from build123d import *

# Parameters (mm, degrees)
SKETCH1_R               = 13
BOSS_EXTRUDE1_DEPTH     = 1
CUT_EXTRUDE2_DEPTH      = 1
FILLET1_R               = 2
SKETCH4_R               = 0.5
CUT_EXTRUDE3_DEPTH      = 1
SKETCH6_R               = 0.85
CUT_EXTRUDE4_DEPTH      = 10
FILLET2_R               = 0.5
BOSS_EXTRUDE4_START     = -1
BOSS_EXTRUDE4_DEPTH     = 1
FILLET4_R               = 0.1
CUT_EXTRUDE6_DEPTH      = 19.411952786
CUT_EXTRUDE6_DEPTH_BACK = 19.411952786
SKETCH11_W              = 6
SKETCH11_H              = 1.5
SKETCH13_R              = 0.325
SKETCH13_W              = 4.85
SKETCH13_H              = 4.4
CUT_EXTRUDE7_DEPTH      = 1


with BuildPart() as part:
    # Sketch1 → Boss-Extrude1 (new body)
    with BuildSketch(Plane(origin=(0, 0, 0), x_dir=(1, 0, 0), z_dir=(0, 1, 0))):
        with Locations(Location((0, 0, 0), (0, 0, 270))):
            Circle(SKETCH1_R)
    extrude(amount=BOSS_EXTRUDE1_DEPTH)

    # Sketch3 → Cut-Extrude2 (cut)
    with BuildSketch(Plane(origin=(0, 0, 0), x_dir=(1, 0, 0), z_dir=(0, 1, 0))):
        with BuildLine():
            Line((-5, -12), (5, -12))
            ThreePointArc((5, -12), (0, -13), (-5, -12))
        make_face()
    extrude(amount=CUT_EXTRUDE2_DEPTH, mode=Mode.SUBTRACT)

    # Fillet1
    fillet1_edges = [part.edges().sort_by_distance(p)[0] for p in [
        (-5, 0.5, 12),
        (5, 0.5, 12),
    ]]
    fillet(fillet1_edges, radius=FILLET1_R)

    # Sketch4 → Cut-Extrude3 (cut)
    with BuildSketch(Plane.XZ):
        with Locations(Location((4.45412, 8.175151, 0), (0, 0, 270))):
            Circle(SKETCH4_R)
        with Locations(Location((-4.61588, 8.175151, 0), (0, 0, 270))):
            Circle(SKETCH4_R)
        with Locations(Location((-7.04588, -8.574849, 0), (0, 0, 270))):
            Circle(SKETCH4_R)
        with Locations(Location((7.74412, -8.574849, 0), (0, 0, 270))):
            Circle(SKETCH4_R)
    extrude(amount=-CUT_EXTRUDE3_DEPTH, mode=Mode.SUBTRACT)

    # Sketch6 → Cut-Extrude4 (cut)
    with BuildSketch(Plane.XZ):
        with Locations((9.958577761, -8.356238926)):
            Circle(SKETCH6_R)
        with Locations((-9.584605379, 8.782672699)):
            Circle(SKETCH6_R)
        with Locations((-9.192388155, -9.192388155)):
            Circle(SKETCH6_R)
        with Locations((10.964088796, 6.984894909)):
            Circle(SKETCH6_R)
    extrude(amount=-CUT_EXTRUDE4_DEPTH, mode=Mode.SUBTRACT)

    # Fillet2
    fillet2_edges = [part.edges().sort_by_distance(p)[0] for p in [
        (10.484191703, 0.5, 7.686463708),
        (11.397112787, 0.5, 6.25346465),
        (-10.138062294, 0.5, 8.137548337),
        (-8.990172858, 0.5, 9.390249836),
        (-8.57201926, 0.5, -9.773458232),
        (-9.773458232, 0.5, -8.57201926),
        (10.483367978, 0.5, -7.687587127),
        (9.39121315, 0.5, -8.989166567),
    ]]
    fillet(fillet2_edges, radius=FILLET2_R)

    # Sketch10 → Boss-Extrude4 (add)
    with BuildSketch(Plane(origin=(0, 1, 0), x_dir=(1, 0, 0), z_dir=(0, 1, 0)).offset(BOSS_EXTRUDE4_START)):
        with BuildLine():
            Line((-6.597998718, -11.201179086), (-6.8517679, -11.631993666))
            ThreePointArc((-6.8517679, -11.631993666), (-7.839489902, -10.990559498), (-8.767548652, -10.265480536))
            Line((-8.767548652, -10.265480536), (-8.442824628, -9.885277553))
            ThreePointArc((-8.442824628, -9.885277553), (-7.549138424, -10.583501739), (-6.597998718, -11.201179086))
        make_face()
        with BuildLine():
            Line((8.442824628, -9.885277553), (8.767548652, -10.265480536))
            ThreePointArc((8.767548652, -10.265480536), (7.839489902, -10.990559498), (6.8517679, -11.631993666))
            Line((6.8517679, -11.631993666), (6.597998718, -11.201179086))
            ThreePointArc((6.597998718, -11.201179086), (7.549138424, -10.583501739), (8.442824628, -9.885277553))
        make_face()
    extrude(amount=BOSS_EXTRUDE4_DEPTH)

    # Fillet4
    fillet4_edges = [part.edges().sort_by_distance(p)[0] for p in [
        (-8.442824628, 0.5, 9.885277553),
        (-6.597998718, 0.5, 11.201179086),
        (-6.8517679, 0.5, 11.631993666),
        (-8.767548652, 0.5, 10.265480536),
        (6.597998718, 0.5, 11.201179086),
        (8.442824628, 0.5, 9.885277553),
        (8.767548652, 0.5, 10.265480536),
        (6.8517679, 0.5, 11.631993666),
    ]]
    fillet(fillet4_edges, radius=FILLET4_R)

    # Sketch11 → Cut-Extrude6 (cut, two sides: drawn at the far end of the back side and taken through both)
    with BuildSketch(Plane(origin=(0, 0, 0), x_dir=(1, 0, 0), z_dir=(0, 1, 0)).offset(-CUT_EXTRUDE6_DEPTH_BACK)):
        with Locations((0, -12)):
            Rectangle(SKETCH11_W, SKETCH11_H)
    extrude(amount=CUT_EXTRUDE6_DEPTH + CUT_EXTRUDE6_DEPTH_BACK, mode=Mode.SUBTRACT)

    # Sketch13 → Cut-Extrude7 (cut)
    with BuildSketch(Plane(origin=(0, 1, 0), x_dir=(1, 0, 0), z_dir=(0, 1, 0))):
        with Locations(Location((10.26011, 4.62025, 0), (0, 0, 270))):
            Circle(SKETCH13_R)
        with Locations(Location((10.26011, 5.89025, 0), (0, 0, 270))):
            Circle(SKETCH13_R)
        with Locations((3.51412, 8.889849)):
            Rectangle(SKETCH13_W, SKETCH13_H)
    extrude(amount=-CUT_EXTRUDE7_DEPTH, mode=Mode.SUBTRACT)


solid = part.part
Source: CAD feature listing. Evaluate the final solid. Frame: model axes, mm. A direction names the side the tool comes from. Round coordinates to 2 decimals unless told otherwise and drop trailing zeros. Write each loop counter-clockwise with the first axis right and the second up, starting at its lowest first coordinate (ties: lowest second). Pieces come first, ordered by that corner, then holes. Notation, with made-up numbers: M -15.5,3.25 L 8.5,3.25 A12 ccw 8.5,20.25 Z; hole C -39.75,31 d4. An arc over 180 degrees is marked long. One line per item, written item: value. Start each with the question number.
Item 1: Mould query, pull axis Z, two halves, no side actions, for faces 4 (the flat face through (0, 1, -1)), 5 (the flat face through (0, 0.5, 11.25)), 6 (the cylindrical face through (-8.967, 0.493, 8.198)), 7 (the cylindrical face through (0.7, 0.49, -12.98)). Classes: pulls with the +Z half, pulls with the -Z half, needs draft (parallel to the pull), parting line crosses it, or undercut.
Item 2: Ray query, L1, parallel to X at y = 0.1, z = 8.5; L2, parallel to X at y = 0.9, z = 8.25; L3, parallel to Z at x = 0, y = 0.2. Return the intervals inside material, ascending. Write a range as from..to.
Item 3: Section query A-A (z = 5.25). Return the cut outline in (x, y).
Item 4: Section query B-B (y = 0.4). State how many separate pieces and enclosed holes the cut face has, plus the area to 3 significant figures.
Item 5: Section query C-C (z = -2.25). Return the cut outline in (x, y).
Item 6: Pin query (flat end, axial travel): pin 1 (0.5 mm diameter, centred on x = 4, y = 0.5, fed in from -Z); pin 2 (0.6 mm diameter, centred on y = 0.5, z = 11.5, fed in from +X). Return the tip coordinate at first contact, or that it passes through.
Item 7: Set-up query: faces 1 (the cylindrical face through (5.963, 0.493, 11.552)), 2 (the flat face through (1.089, 0.5, -8.9)), 3 (the flat face through (0, 0, -1)). Return all of +Z, -Z, +X, -X, +Y, -Y with unobstructed straight access to the full face (end or side cutting, diameter ignored); none if empty.
Result set:
1. face 4: needs draft
1. face 5: pulls with the +Z half
1. face 6: undercut
1. face 7: pulls with the -Z half
2. L1: x = -8.78..-5, -4.24..4.07, 4.83..9.84
2. L2: x = -8.92..-5.11, -4.12..3.96, 4.95..10.05
2. L3: z = -13..11.25
3. outline: M -11.89,0 L 11.89,0 L 11.89,1 L -11.89,1 Z
4. separate pieces: 1
4. enclosed holes: 7
4. area: 492 mm²
5. outline: M -12.8,0 L 12.8,0 L 12.8,1 L -12.8,1 Z
6. pin 1: stops at z = -12.45
6. pin 2: stops at x = 7.54
7. face 1: +Z, +Y, -Y
7. face 2: +Y, -Y
7. face 3: +Z, -Z, +X, -X, -Y
